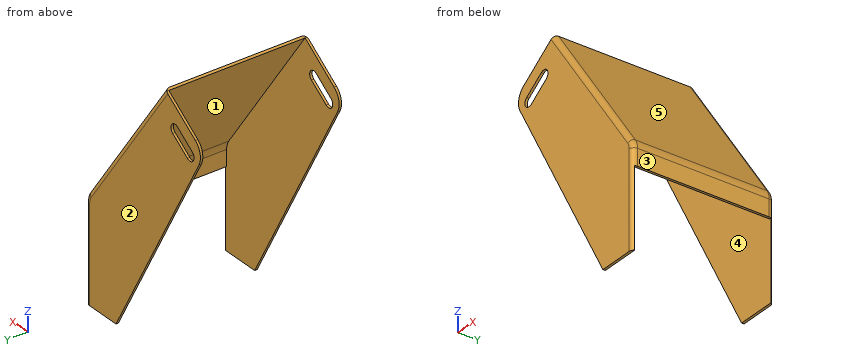
```python
from build123d import *

# Parameters (mm, degrees)
BOSS_EXTRUDE1_DEPTH = 87.5
BOSS_EXTRUDE2_DEPTH = 1.5
FILLET1_R           = 10
FILLET2_R           = 3
CUT_EXTRUDE1_REACH  = 205.273
SKETCH3_W           = 49.374063928
SKETCH3_H           = 85


with BuildPart() as part:
    # Sketch1 → Boss-Extrude1 (new body)
    with BuildSketch(Plane(origin=(0, 0, 0), x_dir=(1, 0, 0), z_dir=(0, 1, 0))):
        Polygon((0, 0), (0, -63), (-65.96129018, -157.202485093), (-67.190018247, -156.342120439), (-1.5, -62.527051817), (-1.5, 0), align=None)
    extrude(amount=BOSS_EXTRUDE1_DEPTH)

    # Sketch2 → Boss-Extrude2 (add)
    with BuildSketch(Plane.XZ):
        with BuildLine():
            Line((0, 0), (-25, 0))
            Line((-25, 0), (-94.410596168, 126.398468668))
            ThreePointArc((-94.410596168, 126.398468668), (-95.384485345, 133.480683165), (-91.38102437, 139.403395594))
            Line((-91.38102437, 139.403395594), (-65.96129018, 157.202485093))
            Line((-65.96129018, 157.202485093), (0, 63))
            Line((0, 63), (0, 0))
        make_face()
        with BuildLine():
            Line((-72.511956454, 134.304040356), (-84.799237119, 125.700393811))
            ThreePointArc((-84.799237119, 125.700393811), (-89.673786801, 126.559908439), (-88.814272173, 131.434458121))
            Line((-88.814272173, 131.434458121), (-76.526991509, 140.038104666))
            ThreePointArc((-76.526991509, 140.038104666), (-71.652441827, 139.178590039), (-72.511956454, 134.304040356))
        make_face(mode=Mode.SUBTRACT)
    boss_extrude2 = extrude(amount=-BOSS_EXTRUDE2_DEPTH)

    # Mirror1: Boss-Extrude2 across plane
    add(boss_extrude2.mirror(Plane.ZX.offset(44)))

    # Fillet1
    fillet1_edges = [part.edges().sort_by_distance(p)[0] for p in [
        (0, 44, 63),
        (-1.5, 44, 62.527051817),
    ]]
    fillet(fillet1_edges, radius=FILLET1_R)

    # Fillet2
    fillet2_edges = [part.edges().sort_by_distance(p)[0] for p in [
        (0, 88, 29.923506056),
        (-33.884884869, 0, 111.392630784),
        (0, 0, 29.923506056),
        (-0.462830493, 0, 62.854070106),
        (-33.884884869, 88, 111.392630784),
        (-0.462830493, 88, 62.854070106),
    ]]
    fillet(fillet2_edges, radius=FILLET2_R)

    # Cut-Extrude1: up to this face of the body (flat: up to its plane)
    cut_extrude1_end = Plane(part.part.faces().sort_by_distance((0, 44, 29.923506056))[0])
    # Sketch3 → Cut-Extrude1 (cut, up to the picked face)
    with BuildSketch(Plane.ZY.offset(1.5), mode=Mode.PRIVATE) as cut_extrude1_sk1:
        with Locations((24.687031964, 44)):
            Rectangle(SKETCH3_W, SKETCH3_H)
    cut_extrude1_tool1 = split(extrude(cut_extrude1_sk1.sketch, amount=-CUT_EXTRUDE1_REACH, mode=Mode.PRIVATE), bisect_by=cut_extrude1_end, keep=Keep.BOTH, mode=Mode.PRIVATE)
    add(cut_extrude1_tool1.solids().sort_by(Axis((-1.5, 44, 24.687032), (1, 0, 0)))[0], mode=Mode.SUBTRACT)


solid = part.part
```
Source: CAD feature listing. Evaluate the final solid. Frame: model axes, mm. Face numbers are marked on the shaded views. A direction names the side the tool comes from. Coordinates: 2 decimals unless noted, no trailing zeros. Loops run counter-clockwise (first coordinate to the right, second up) from the corner with the lowest first, then second, coordinate; pieces in that order, holes last. Notation, with made-up numbers: (59.5, 16) -> (118.5, 16) arc R13 ccw to (118.5, 35) -> close; hole circle Ø6 at (28.5, -34.75). An arc over 180 degrees is marked (long way). One line per item, written item: value. Start each with the question number.
Q1. Mould query, pull axis Y, two halves, no side actions, for the marked faces 1, 2 and 3. Classes: pulls with the +Y half, pulls with the -Y half, needs draft (parallel to the pull), parting line crosses it, or undercut.
Q2. Set-up query: the marked faces 4 and 5. Return all of +Z, -Z, +X, -X, +Y, -Y with unobstructed straight access to the full face (end or side cutting, diameter ignored); none if empty.
Q3. Section query C-C, the plane y = 7. Return the cut outline in (x, z).
Q4. Section query A-A, the plane z = 18.5. Return the cut outline in (x, y).
Q5. Section query D-D, the plane z = 45. Return the cut outline in (x, y).
Q6. Line query: line 1 along Y through (x, z) = (-55.5, 135); line 2 along X through (y, z) = (57.5, 59); line 3 along Z through (x, y) = (-25, 69). Output: solid intervals per line, ascending.
Q7. Contact query for flat-ended pins moving along their axis: P1, Ø2, axis at y = 45.5, z = 131.5, coming from the -X side; P2, Ø1.2, axis at x = -0.5, y = 28, coming from the -Z side; P3, Ø8, axis at x = -29, z = 107, coming from the +Y side. Output: stop coordinate, or through.
Q8. Section query B-B, the plane x = -81.5. Return the cut outline in (y, z).
Results:
1. face 1: undercut
1. face 2: pulls with the +Y half
1. face 3: needs draft
2. face 4: -Z, -X
2. face 5: +Z, +X, +Y, -Y
3. outline: (-67.19, 156.34) -> (-3.31, 65.11) arc R10 cw to (-1.5, 59.37) -> (-1.5, 49.37) -> (0, 49.37) -> (0, 59.85) arc R10 ccw to (-1.81, 65.58) -> (-65.96, 157.2) -> close
4. outline: (-35.16, 0) -> (-3, 0) arc R3 ccw to (-0.4, 1.5) -> (-35.16, 1.5) -> close; (-35.16, 86.5) -> (-0.4, 86.5) arc R3 ccw to (-3, 88) -> (-35.16, 88) -> close
5. outline: (-49.71, 0) -> (-3, 0) arc R3 ccw to (-0.4, 1.5) -> (-49.71, 1.5) -> close; (-49.71, 86.5) -> (-0.4, 86.5) arc R3 ccw to (-3, 88) -> (-49.71, 88) -> close
6. line 1: 0 to 1.5, 86.5 to 88
6. line 2: -1.5 to 0
6. line 3: 96.09 to 98.7
7. P1: x = -50.5
7. P2: z = 49.37
7. P3: y = 87.96
8. outline: (0, 102.89) -> (1.5, 102.89) -> (1.5, 128.01) -> (0, 128.01) -> close; (0, 136.56) -> (1.5, 136.56) -> (1.5, 146.32) -> (0, 146.32) -> close; (86.5, 102.89) -> (88, 102.89) -> (88, 128.01) -> (86.5, 128.01) -> close; (86.5, 136.56) -> (88, 136.56) -> (88, 146.32) -> (86.5, 146.32) -> close
